```python
from build123d import *

# Parameters (mm, degrees)
F0_W     = 1.2
F0_H     = 0.3
F1_DEPTH = 4.7
F3_DEPTH = 1.05
F6_DEPTH = 2
F7_SIZE  = 1


with BuildPart() as f1:
    # F0 (on Front) → F1 (new body)
    with BuildSketch(Plane.XZ):
        with BuildLine():
            Line((0, 31.15), (0, 0))
            Line((0, 0), (19.75, 0))
            Line((19.75, 0), (19.75, 31.15))
            Line((19.75, 31.15), (18.55, 31.15))
            Line((18.55, 31.15), (10.275, 31.15))
            Line((10.275, 31.15), (10.275, 31.45))
            Line((10.275, 31.45), (18.55, 31.45))
            Line((18.55, 31.45), (19.75, 31.45))
            Line((19.75, 31.45), (19.75, 52.5))
            Line((19.75, 52.5), (19.75, 55.1716775767))
            ThreePointArc((19.75, 55.1716775767), (18.375, 59.5), (19.75, 63.8283224233))
            Line((19.75, 63.8283224233), (19.75, 65))
            Line((19.75, 65), (0, 65))
            Line((0, 65), (0, 63.8283224233))
            ThreePointArc((0, 63.8283224233), (1.0229892277, 61.7707377656), (1.375, 59.5))
            ThreePointArc((1.375, 59.5), (1.0229892277, 57.2292622344), (0, 55.1716775767))
            Line((0, 55.1716775767), (0, 52.5))
            Line((0, 52.5), (0, 31.45))
            Line((0, 31.45), (1.2, 31.45))
            Line((1.2, 31.45), (9.475, 31.45))
            Line((9.475, 31.45), (9.475, 31.15))
            Line((9.475, 31.15), (1.2, 31.15))
            Line((1.2, 31.15), (0, 31.15))
        make_face()
        with BuildLine():
            Line((-2, 52.5), (0, 52.5))
            Line((0, 52.5), (0, 55.1716775767))
            ThreePointArc((0, 55.1716775767), (-0.9094386331, 54.1103878035), (-2, 53.2362650918))
            Line((-2, 53.2362650918), (-2, 52.5))
        make_face()
        with BuildLine():
            Line((19.75, 55.1716775767), (19.75, 52.5))
            Line((19.75, 52.5), (21.75, 52.5))
            Line((21.75, 52.5), (21.75, 53.2362650918))
            ThreePointArc((21.75, 53.2362650918), (20.6594386331, 54.1103878035), (19.75, 55.1716775767))
        make_face()
        with Locations((0.6, 31.3)):
            Rectangle(F0_W, F0_H)
        with Locations((19.15, 31.3)):
            Rectangle(F0_W, F0_H)
    extrude(amount=F1_DEPTH)

    # F2 (on face) → F3 (cut)
    with BuildSketch(Plane.XZ.offset(4.7)):
        Polygon((13.475, 37.5), (6.275, 37.5), (6.275, 2.2), (6.275, 0), (13.475, 0), (13.475, 2.2), align=None)
    extrude(amount=-F3_DEPTH, mode=Mode.SUBTRACT)

    # F5 (on face) → F6 (join)
    with BuildSketch(Plane.XZ.offset(4.7)):
        with BuildLine():
            Line((-2, 52.5), (0, 52.5))
            Line((0, 52.5), (19.75, 52.5))
            Line((19.75, 52.5), (21.75, 52.5))
            Line((21.75, 52.5), (21.75, 53.2362650918))
            ThreePointArc((21.75, 53.2362650918), (18.5052276407, 58.1084342015), (19.75, 63.8283224233))
            Line((19.75, 63.8283224233), (19.75, 65))
            Line((19.75, 65), (0, 65))
            Line((0, 65), (0, 63.8283224233))
            ThreePointArc((0, 63.8283224233), (1.2447723593, 58.1084342015), (-2, 53.2362650918))
            Line((-2, 53.2362650918), (-2, 52.5))
        make_face()
    extrude(amount=F6_DEPTH)

    # F7
    f7_edges = [f1.edges().sort_by_distance(p)[0] for p in [
        (0, -2.35, 0),
        (19.75, -2.35, 0),
        (3.1375, -4.7, 0),
        (16.6125, -4.7, 0),
        (9.875, -3.65, 0),
    ]]
    chamfer(f7_edges, length=F7_SIZE)


solid = f1.part
```
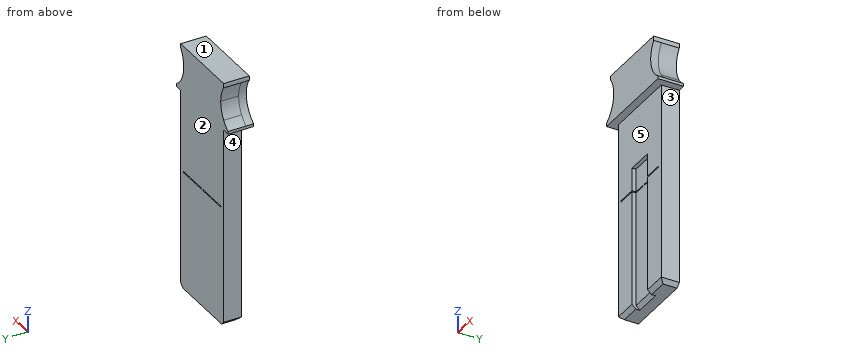
The listing builds one solid part. Answer for the finished solid, in the listing's coordinates (mm). Face numbers are marked on the shaded views. A direction names the side the tool comes from. Give positions to 0.01 mm unless a question says otherwise; leave off trailing zeros. Order: outer loops, then holes, each group sorted by start corner. A loop starts at its lowest first (then second) coordinate and runs counter-clockwise, first axis right, second up. Notation, with made-up numbers: (-30, 70.25) -> (-15, 70.25) arc R24 ccw to (-15, 90.25) -> close; hole circle Ø5 at (3, 1.5). An arc over 180 degrees is marked (long way). Write each question's results on one line, items separated by ' | '.
Q1. The part is cut by section B-B, the plane x = 11. Give the vertices of the cut face in (y, z), and give its area (3 significant figures).
Checked values:
outline: (-6.7, 52.5) -> (-4.7, 52.5) -> (-4.7, 37.5) -> (-3.65, 37.5) -> (-3.65, 31.45) -> (0, 31.45) -> (0, 65) -> (-6.7, 65) -> close; (-3.65, 1) -> (-2.65, 0) -> (0, 0) -> (0, 31.15) -> (-3.65, 31.15) -> close | area: 290 mm^2
Q2. The part is cut by section D-D, the plane x = 3. Give the vertices of the cut face in (y, z), and give its area (3 significant figures).
Checked values:
outline: (-6.7, 52.5) -> (-4.7, 52.5) -> (-4.7, 31.45) -> (0, 31.45) -> (0, 65) -> (-6.7, 65) -> close; (-4.7, 1) -> (-3.7, 0) -> (0, 0) -> (0, 31.15) -> (-4.7, 31.15) -> close | area: 329 mm^2
Q3. The part is cut by section C-C, the plane z = 28.5. Give the vertices of the cut face in (x, y) (3 decimals), and give its area (3 significant figures).
Checked values:
outline: (0, -4.7) -> (6.275, -4.7) -> (6.275, -3.65) -> (13.475, -3.65) -> (13.475, -4.7) -> (19.75, -4.7) -> (19.75, 0) -> (0, 0) -> close | area: 85.3 mm^2
Q4. Each of these flat-tipped pins is pushed along its axis until it touches: P1, Ø1, axis at x = 17.5, z = 24, coming from the -Y side; P2, Ø0.6, axis at y = -4, z = 64.5, coming from the +X side; P3, Ø1.6, axis at y = -4, z = 8.5, coming from the -X side. Where does it stop, or does it pass through?
Checked values:
P1: stops at y = -4.7 | P2: stops at x = 19.75 | P3: stops at x = 0
Q5. Straight lines are drawn through the part: probe 1 along X at (y, z) = (-4.5, 17) (3 decimals); probe 2 along Z at (x, y) = (6.75, -5.5); probe 3 along X at (y, z) = (-1.5, 29). For each, find the intervals that lie inside material, in ascending order. Write a range as from..to.
Checked values:
probe 1: x = 0..6.275, 13.475..19.75 | probe 2: z = 52.5..65 | probe 3: x = 0..19.75
Q6. Which of the six approach directions +Z, -Z, +X, -X, +Y, -Y give full straight-line access (tool end or side, diameter ignored) to the marked faces 1, 2, 3, 4 and 5?
Checked values:
face 1: +Z, +X, -X, +Y, -Y | face 2: +Z, -Z, +X, -X, +Y | face 3: -Z, +X, +Y, -Y | face 4: -Z, -X, +Y, -Y | face 5: -Z, +X, -X, -Y
Q7. The part is cut by section A-A, the plane y = -1.5. Give the vertices of the cut face in (x, z) (3 decimals), and give its area (3 significant figures).
Checked values:
outline: (-2, 52.5) -> (0, 52.5) -> (0, 1) -> (1, 0) -> (18.75, 0) -> (19.75, 1) -> (19.75, 52.5) -> (21.75, 52.5) -> (21.75, 53.236) arc R7.5 cw to (19.75, 63.828) -> (19.75, 65) -> (0, 65) -> (0, 63.828) arc R7.5 cw to (-2, 53.236) -> close; hole (1.2, 31.15) -> (9.475, 31.15) -> (9.475, 31.45) -> (1.2, 31.45) -> close; hole (10.275, 31.15) -> (18.55, 31.15) -> (18.55, 31.45) -> (10.275, 31.45) -> close | area: 1,270 mm^2
